Verification items for the finished model (mm, model axes). Face numbers are marked on the shaded views. A direction names the side the tool comes from. Coordinates: 2 decimals unless noted, no trailing zeros. Order: outer loops, then holes, each group sorted by start corner. A loop starts at its lowest first (then second) coordinate and runs counter-clockwise, first axis right, second up. Notation, with made-up numbers: M 56.5,62 L 100.5,62 A11 ccw 100.5,82 Z; hole C -22,-32 d1. An arc over 180 degrees is marked long. Answer as a JSON object with one key per item and string values. Group by question number.
(1) Material ranges on line 1 (Z direction, x = -16, y = -11); line 2 (Y direction, x = -7, z = -6.5); line 3 (Z direction, x = -16.5, y = 11), recorded low to high.
(2) Gauge pin test, flat ends, axial feed: pin 1 Ø2 at (x, y) = (9, -2.5) entering from +Z; pin 2 Ø2 at (y, z) = (-1, 13.5) entering from -X; pin 3 Ø19 at (x, y) = (-0.5, 8) entering from -Z; pin 4 Ø2 at (y, z) = (-15.5, -24.5) entering from +X. Record the tip position at first contact, or that the pin passes through.
(3) Cross-section at C-C (z = 18.5). Enter the section's corners in (x, y).
(4) Cross-section at A-A (y = 0). Enter the section's corners in (x, z).
(5) Access from +Z, -Z, +X, -X, +Y, -Y to the whole of each face (thin tool, end or side, straight path). Record for the marked faces 1 and 2.
(6) Mould release check, pull along X, two halves, no side actions. Record for the marked faces 3, 4, 5 and 6: released by +X, released by -X, zero draft, split by the parting line, or undercut.
(7) Cross-section at D-D (z = -43). Enter the section's corners in (x, y).
(8) Cross-section at B-B (z = -4.5). Enter the section's corners in (x, y).
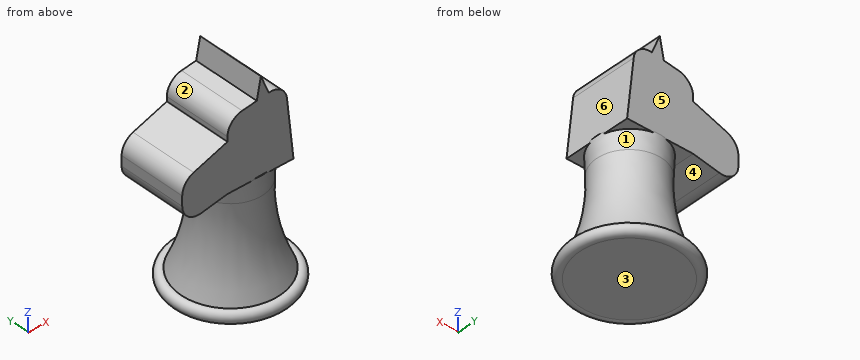
from build123d import *

# Parameters (mm, degrees)
F3_DEPTH = 12.7
F4_DEPTH = 12.7


with BuildPart() as f1:
    # F0 (on Front) → F1 (revolve)
    with BuildSketch(Plane.XZ):
        with BuildLine():
            Line((-19.05, -50.974112), (0, -50.974112))
            Line((0, -50.974112), (0, -6.467288))
            Line((0, -6.467288), (-12.921196, -6.467288))
            Line((-12.921196, -6.467288), (-12.582219, -14.195322))
            ThreePointArc((-12.582219, -14.195322), (-13.853409, -30.877259), (-19.05, -46.780039))
            ThreePointArc((-19.05, -46.780039), (-22.088268, -48.877075), (-19.05, -50.974112))
        make_face()
    revolve(axis=Axis((0, 0, -22.399112), (0, 0, 1)))

    # F2 (on Front) → F3 (join)
    with BuildSketch(Plane.XZ):
        with BuildLine():
            Line((-12.884437, -6.452419), (12.582218, -7.097661))
            Line((12.582218, -7.097661), (10.049637, 15.948844))
            ThreePointArc((10.049637, 15.948844), (7.710426, 20.208945), (3.044008, 21.56722))
            Line((3.044008, 21.56722), (-1.583988, 21.05865))
            Line((-1.583988, 21.05865), (-7.228063, 20.438422))
            ThreePointArc((-7.228063, 20.438422), (-11.263444, 18.364223), (-12.884437, 14.126419))
            Line((-12.884437, 14.126419), (-12.884437, 12.306017))
            Line((-12.884437, 12.306017), (-12.884437, -6.452419))
        make_face()
        with BuildLine():
            Line((-23.013249, -8.006668), (-12.884437, -6.452419))
            Line((-12.884437, -6.452419), (-12.884437, 12.306017))
            Line((-12.884437, 12.306017), (-25.925016, 8.101342))
            ThreePointArc((-25.925016, 8.101342), (-29.109421, 5.795949), (-30.326372, 2.057726))
            Line((-30.326372, 2.057726), (-30.326372, -1.730133))
            ThreePointArc((-30.326372, -1.730133), (-28.11199, -6.54876), (-23.013249, -8.006668))
        make_face()
        Polygon((-1.583988, 21.05865), (3.044008, 21.56722), (0, 29.035889), align=None)
    extrude(amount=F3_DEPTH)

    # F2 (on Front) → F4 (join)
    with BuildSketch(Plane.XZ):
        with BuildLine():
            Line((-12.884437, -6.452419), (12.582218, -7.097661))
            Line((12.582218, -7.097661), (10.049637, 15.948844))
            ThreePointArc((10.049637, 15.948844), (7.710426, 20.208945), (3.044008, 21.56722))
            Line((3.044008, 21.56722), (-1.583988, 21.05865))
            Line((-1.583988, 21.05865), (-7.228063, 20.438422))
            ThreePointArc((-7.228063, 20.438422), (-11.263444, 18.364223), (-12.884437, 14.126419))
            Line((-12.884437, 14.126419), (-12.884437, 12.306017))
            Line((-12.884437, 12.306017), (-12.884437, -6.452419))
        make_face()
        with BuildLine():
            Line((-23.013249, -8.006668), (-12.884437, -6.452419))
            Line((-12.884437, -6.452419), (-12.884437, 12.306017))
            Line((-12.884437, 12.306017), (-25.925016, 8.101342))
            ThreePointArc((-25.925016, 8.101342), (-29.109421, 5.795949), (-30.326372, 2.057726))
            Line((-30.326372, 2.057726), (-30.326372, -1.730133))
            ThreePointArc((-30.326372, -1.730133), (-28.11199, -6.54876), (-23.013249, -8.006668))
        make_face()
        Polygon((-1.583988, 21.05865), (3.044008, 21.56722), (0, 29.035889), align=None)
    extrude(amount=-F4_DEPTH)


solid = f1.part
Taken from the geometry:
{
 "1": {"line 1": "z = -51.08 to -46.68, -6.93 to 11.3", "line 2": "y = -12.7 to 12.7", "line 3": "z = -51.12 to -46.63, -7.01 to 11.14"},
 "2": {"pin 1": "stops at z = 19.96", "pin 2": "stops at x = -12.88", "pin 3": "stops at z = -50.97", "pin 4": "passes through"},
 "3": {"outline": "M -11.14,-12.7 L 9.2,-12.7 L 9.2,12.7 L -11.14,12.7 Z"},
 "4": {"outline": "M -30.33,-1.73 A6.35 ccw -23.01,-8.01 L -12.88,-6.45 L -12.3,-6.47 L -12.92,-6.47 L -12.58,-14.2 A69.94 cw -19.05,-46.78 A2.24 ccw long -19.05,-50.97 L 19.05,-50.97 A2.24 ccw long 19.05,-46.78 A69.94 cw 12.58,-14.2 L 12.92,-6.47 L 12.51,-6.47 L 10.05,15.95 A6.35 ccw 3.04,21.57 L 0,29.04 L -1.58,21.06 L -7.23,20.44 A6.35 ccw -12.88,14.13 L -12.88,12.31 L -25.93,8.1 A6.35 ccw -30.33,2.06 Z"},
 "5": {"face 1": "none", "face 2": "+Z, -X, +Y, -Y"},
 "6": {"face 3": "undercut", "face 4": "undercut", "face 5": "zero draft", "face 6": "released by +X"},
 "7": {"outline": "C 0,0 d34.85"},
 "8": {"outline": "M -29.69,-12.7 L 12.3,-12.7 L 12.3,12.7 L -29.69,12.7 Z"}
}
